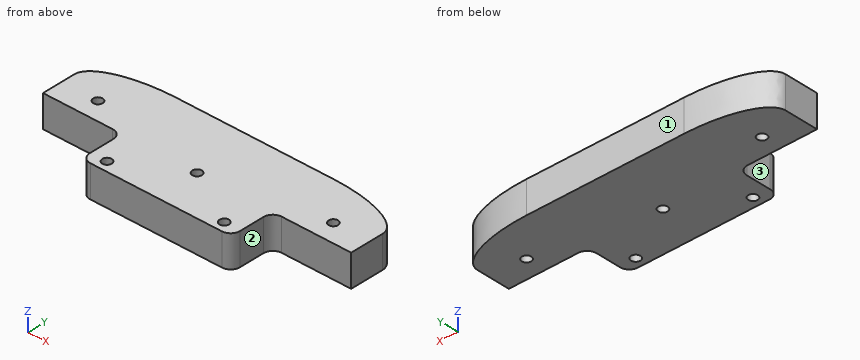
from build123d import *

# Parameters (mm, degrees)
SKETCH_1_R      = 2.5
EXTRUDE_1_DEPTH = 17
FILLET_1_SIZE   = 15
FILLET_1_SIZE_2 = 40
FILLET_2_R      = 5


with BuildPart() as part:
    # 草图1 → 凸台-拉伸1 (new body)
    with BuildSketch(Plane.XY):
        Polygon((-80, 0), (0, 0), (0, 23.4), (42, 23.4), (42, 56.39), (-122, 56.39), (-122, 23.4), (-80, 23.4), align=None)
        with Locations((-40, 23.4)):
            Circle(SKETCH_1_R, mode=Mode.SUBTRACT)
        with Locations((-71.2, 5.4)):
            Circle(SKETCH_1_R, mode=Mode.SUBTRACT)
        with Locations((-8.8, 5.4)):
            Circle(SKETCH_1_R, mode=Mode.SUBTRACT)
        with Locations((-102.6, 34)):
            Circle(SKETCH_1_R, mode=Mode.SUBTRACT)
        with Locations((22.705, 34)):
            Circle(SKETCH_1_R, mode=Mode.SUBTRACT)
    extrude(amount=EXTRUDE_1_DEPTH)

    # 圆角1
    # an asymmetric fillet: 40, 15 mm, written as the material it takes off along each edge
    with BuildSketch(Plane(origin=(42, 56.39, -100), x_dir=(0, -1, 0), z_dir=(0, 0, 1))) as fillet_1_piece_1:
        with BuildLine():
            Bezier((FILLET_1_SIZE, 0), (0, 0), (0, -FILLET_1_SIZE_2), weights=[1, 0.707106781, 1])
            Line((0, -FILLET_1_SIZE_2), (0, 0))
            Line((0, 0), (FILLET_1_SIZE, 0))
        make_face()
    extrude(amount=217, mode=Mode.SUBTRACT)
    with BuildSketch(Plane(origin=(-122, 56.39, -100), x_dir=(1, 0, 0), z_dir=(0, 0, 1))) as fillet_1_piece_2:
        with BuildLine():
            Bezier((FILLET_1_SIZE_2, 0), (0, 0), (0, -FILLET_1_SIZE), weights=[1, 0.707106781, 1])
            Line((0, -FILLET_1_SIZE), (0, 0))
            Line((0, 0), (FILLET_1_SIZE_2, 0))
        make_face()
    extrude(amount=217, mode=Mode.SUBTRACT)

    # 圆角2
    fillet_2_edges = [part.edges().sort_by_distance(p)[0] for p in [
        (0, 0, 8.5),
        (-80, 0, 8.5),
        (-80, 23.4, 8.5),
        (0, 23.4, 8.5),
    ]]
    fillet(fillet_2_edges, radius=FILLET_2_R)


solid = part.part
Build history of the part. All positions in model axes, mm. Face numbers are marked on the shaded views. A direction names the side the tool comes from. Round coordinates to 2 decimals unless told otherwise and drop trailing zeros. Loops run counter-clockwise (first coordinate to the right, second up) from the corner with the lowest first, then second, coordinate; pieces in that order, holes last. Notation, with made-up numbers: (-23.5, 22.25) -> (4.5, 22.25) arc R20 cw to (4.5, 50.25) -> close; hole circle Ø7 at (-3, -37.75). An arc over 180 degrees is marked (long way). Use CSV: the item, a comma, the result in double quotes. Start each with the question number.
Q1. Flat gauge pins, fed straight in: pin 1 Ø1.5 at (y, z) = (46, 10) entering from -X; pin 2 Ø8 at (x, y) = (-102.6, 34) entering from +Z; pin 3 Ø4 at (y, z) = (16, 8.5) entering from -X; pin 4 Ø8.5 at (x, z) = (-106, 9) entering from -Y. Where does each tip first touch, or does it go through?
Q2. Drill centre lines: L1, parallel to Y at x = -71.2, z = 12.75; L2, parallel to X at y = 23.5, z = 8.25; L3, parallel to X at y = 4, z = 12. Where is each one in solid material? Low to high.
Q3. Saw through at B-B on y = 34. Give the cut face in (x, z) (3 decimals), and give its area (3 significant figures).
Q4. Saw through at C-C on z = 3.5. Count the separate pieces of the cut face and the enclosed holes in it, and give its area (3 significant figures).
Q5. Which spindle directions (+Z, -Z, +X, -X, +Y, -Y) get a long thin tool onto all of the face, cutting with end or side? Do the marked faces 1, 2 and 3. Say none if no direction does.
Q6. Saw through at A-A on x = -8.8. Give the cut face in (y, z).
Solutions:
1,pin 1,"stops at x = -120.65"
1,pin 2,"stops at z = 17"
1,pin 3,"stops at x = -80"
1,pin 4,"stops at y = 23.4"
2,L1,"y = 0 to 2.9, 7.9 to 56.39"
2,L2,"x = -122 to -42.5, -37.5 to 42"
2,L3,"x = -79.9 to -73.27, -69.13 to -10.87, -6.73 to -0.1"
3,outline,"(-122, 0) -> (-105.1, 0) -> (-105.1, 17) -> (-122, 17) -> close; (-100.1, 0) -> (20.205, 0) -> (20.205, 17) -> (-100.1, 17) -> close; (25.205, 0) -> (42, 0) -> (42, 17) -> (25.205, 17) -> close"
3,area,"2,620 mm^2"
4,separate pieces,"1"
4,enclosed holes,"5"
4,area,"6,930 mm^2"
5,face 1,"+Z, -Z, +X, -X, +Y"
5,face 2,"+Z, -Z, +X, -Y"
5,face 3,"+Z, -Z, -X, -Y"
6,outline,"(0, 0) -> (2.9, 0) -> (2.9, 17) -> (0, 17) -> close; (7.9, 0) -> (56.39, 0) -> (56.39, 17) -> (7.9, 17) -> close"
